Can you work these out from the model? Positions are in its coordinate system, mm. Give positions to 0.01 mm unless a question says otherwise; leave off trailing zeros. Write each loop counter-clockwise with the first axis right and the second up, starting at its lowest first coordinate (ties: lowest second). Pieces come first, ordered by that corner, then holes. Notation, with made-up numbers: M 18,47.5 L 66,47.5 A20 cw 66,78.5 Z; hole C 73,86.25 d11. An arc over 180 degrees is marked long. Answer as CSV lines item,"result". Start each with the question number.
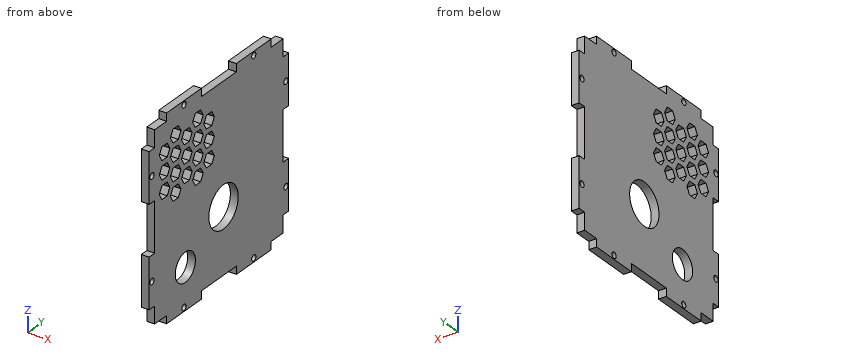
```python
from build123d import *

# Parameters (mm, degrees)
CROQUIS1_W                 = 70
CROQUIS1_H                 = 70
SALIENTE_EXTRUIR1_DEPTH    = 1.5
CROQUIS2_W                 = 19
CROQUIS2_H                 = 3
CROQUIS2_R                 = 1.15
SALIENTE_EXTRUIR2_DEPTH    = 1.5
MATRIZL1_COUNT             = 2
MATRIZL1_PITCH             = 38
SIMETR_A1_COPY_1_SKETCH_W  = 19
SIMETR_A1_COPY_1_SKETCH_H  = 3
SIMETR_A1_COPY_1_SKETCH_R  = 1.15
SIMETR_A1_COPY_1_DEPTH     = 1.5
CROQUIS5_W                 = 3
CROQUIS5_H                 = 19
CROQUIS5_R                 = 1.15
SALIENTE_EXTRUIR3_DEPTH    = 1.5
MATRIZL2_COUNT             = 2
MATRIZL2_PITCH             = 38
SIMETR_A2_COPY_1_SKETCH_W  = 3
SIMETR_A2_COPY_1_SKETCH_H  = 19
SIMETR_A2_COPY_1_SKETCH_R  = 1.15
SIMETR_A2_COPY_1_DEPTH     = 1.5
CORTAR_EXTRUIR2_DEPTH      = 54.761045377
CORTAR_EXTRUIR2_DEPTH_BACK = 54.761045377
CROQUIS4_R                 = 5.5
CORTAR_EXTRUIR3_DEPTH      = 54.761045377
CORTAR_EXTRUIR3_DEPTH_BACK = 54.761045377
CROQUIS6_R                 = 8
CORTAR_EXTRUIR7_DEPTH      = 54.761045377
CORTAR_EXTRUIR7_DEPTH_BACK = 54.761045377
PATR_N_START               = -1.5
PATR_N_DE_RAYADO3_DEPTH    = 3


# Read off the part's stored shape, not the designer's step: Patrón de rayado3
with BuildPart() as part:
    # Croquis1 → Saliente-Extruir1 (new, symmetric)
    with BuildSketch(Plane(origin=(0, 0, 0), x_dir=(0, 0, -1), z_dir=(1, 0, 0))):
        Rectangle(CROQUIS1_W, CROQUIS1_H)
    extrude(amount=SALIENTE_EXTRUIR1_DEPTH, both=True)

    # Croquis2 → Saliente-Extruir2 (add, symmetric)
    with BuildSketch(Plane(origin=(0, 0, 0), x_dir=(0, 0, -1), z_dir=(1, 0, 0))):
        with Locations((-19, 36.5)):
            Rectangle(CROQUIS2_W, CROQUIS2_H)
        with Locations((-19, 36.5)):
            Circle(CROQUIS2_R, mode=Mode.SUBTRACT)
    saliente_extruir2 = extrude(amount=SALIENTE_EXTRUIR2_DEPTH, both=True)

    # MatrizL1: Saliente-Extruir2 ×2
    with Locations(*[(0, 0, -i * MATRIZL1_PITCH) for i in range(1, MATRIZL1_COUNT)]):
        add(saliente_extruir2)

    # Simetría1: Saliente-Extruir2 across plane
    add(saliente_extruir2.mirror(Plane.ZX))

    # Simetría1 copy 1 sketch → Simetría1 copy 1 (add, symmetric)
    with BuildSketch(Plane(origin=(0, 0, -38), x_dir=(0, 0, -1), z_dir=(1, 0, 0))):
        with Locations((-19, -36.5)):
            Rectangle(SIMETR_A1_COPY_1_SKETCH_W, SIMETR_A1_COPY_1_SKETCH_H)
        with Locations((-19, -36.5)):
            Circle(SIMETR_A1_COPY_1_SKETCH_R, mode=Mode.SUBTRACT)
    extrude(amount=SIMETR_A1_COPY_1_DEPTH, both=True)

    # Croquis5 → Saliente-Extruir3 (add, symmetric)
    with BuildSketch(Plane(origin=(0, 0, 0), x_dir=(0, 0, -1), z_dir=(1, 0, 0))):
        with Locations((-36.5, 19)):
            Rectangle(CROQUIS5_W, CROQUIS5_H)
        with Locations((-36.5, 19)):
            Circle(CROQUIS5_R, mode=Mode.SUBTRACT)
    saliente_extruir3 = extrude(amount=SALIENTE_EXTRUIR3_DEPTH, both=True)

    # MatrizL2: Saliente-Extruir3 ×2
    with Locations(*[(0, -i * MATRIZL2_PITCH, 0) for i in range(1, MATRIZL2_COUNT)]):
        add(saliente_extruir3)

    # Simetría2: Saliente-Extruir3 across plane
    add(saliente_extruir3.mirror(Plane.XY))

    # Simetría2 copy 1 sketch → Simetría2 copy 1 (add, symmetric)
    with BuildSketch(Plane(origin=(0, -38, 0), x_dir=(0, 0, 1), z_dir=(1, 0, 0))):
        with Locations((-36.5, -19)):
            Rectangle(SIMETR_A2_COPY_1_SKETCH_W, SIMETR_A2_COPY_1_SKETCH_H)
        with Locations((-36.5, -19)):
            Circle(SIMETR_A2_COPY_1_SKETCH_R, mode=Mode.SUBTRACT)
    extrude(amount=SIMETR_A2_COPY_1_DEPTH, both=True)

    # Croquis4 → Cortar-Extruir2 (cut, two sides: drawn at the far end of the back side and taken through both)
    with BuildSketch(Plane(origin=(0, 0, 0), x_dir=(0, 0, -1), z_dir=(1, 0, 0)).offset(-CORTAR_EXTRUIR2_DEPTH_BACK)):
        with Locations((22.355, -18.3)):
            Circle(CROQUIS4_R)
    extrude(amount=CORTAR_EXTRUIR2_DEPTH + CORTAR_EXTRUIR2_DEPTH_BACK, mode=Mode.SUBTRACT)

    # Croquis6 → Cortar-Extruir3 (cut, two sides: drawn at the far end of the back side and taken through both)
    with BuildSketch(Plane(origin=(0, 0, 0), x_dir=(0, 0, -1), z_dir=(1, 0, 0)).offset(-CORTAR_EXTRUIR3_DEPTH_BACK)):
        with Locations((10.355, 2.5)):
            Circle(CROQUIS6_R)
    extrude(amount=CORTAR_EXTRUIR3_DEPTH + CORTAR_EXTRUIR3_DEPTH_BACK, mode=Mode.SUBTRACT)

    # Croquis11 → Cortar-Extruir7 (cut, two sides: drawn at the far end of the back side and taken through both)
    with BuildSketch(Plane(origin=(0, 0, 0), x_dir=(0, 0, -1), z_dir=(1, 0, 0)).offset(-CORTAR_EXTRUIR7_DEPTH_BACK)):
        Polygon((-20, -16.056624327), (-20, -18.943375673), (-17.5, -20.386751346), (-15, -18.943375673), (-15, -16.056624327), (-17.5, -14.613248654), align=None)
    extrude(amount=CORTAR_EXTRUIR7_DEPTH + CORTAR_EXTRUIR7_DEPTH_BACK, mode=Mode.SUBTRACT)

    # Patrón de rayado3 outline → Patrón de rayado3 (cut)
    with BuildSketch(Plane.YZ.offset(PATR_N_START)):
        Polygon((-20.675426481, 7), (-22.118802154, 9.5), (-25.005553499, 9.5), (-26.448929172, 7), (-25.005553499, 4.5), (-22.118802154, 4.5), align=None)
        Polygon((-8.551070828, 7), (-9.994446501, 9.5), (-12.881197846, 9.5), (-14.324573519, 7), (-12.881197846, 4.5), (-9.994446501, 4.5), align=None)
        Polygon((-22.118802154, 25.5), (-20.675426481, 28), (-22.118802154, 30.5), (-25.005553499, 30.5), (-26.448929172, 28), (-25.005553499, 25.5), align=None)
        Polygon((-12.881197846, 25.5), (-9.994446501, 25.5), (-8.551070828, 28), (-9.994446501, 30.5), (-12.881197846, 30.5), (-14.324573519, 28), align=None)
        Polygon((-32.511106999, 17.5), (-31.067731326, 15), (-28.18097998, 15), (-26.737604307, 17.5), (-28.18097998, 20), (-31.067731326, 20), align=None)
        Polygon((-8.262395693, 17.5), (-6.81902002, 15), (-3.932268674, 15), (-2.488893001, 17.5), (-3.932268674, 20), (-6.81902002, 20), align=None)
        Polygon((-16.056624327, 8), (-14.613248654, 10.5), (-16.056624327, 13), (-18.943375673, 13), (-20.386751346, 10.5), (-18.943375673, 8), align=None)
        Polygon((-22.118802154, 18.5), (-20.675426481, 21), (-22.118802154, 23.5), (-25.005553499, 23.5), (-26.448929172, 21), (-25.005553499, 18.5), align=None)
        Polygon((-12.881197846, 18.5), (-9.994446501, 18.5), (-8.551070828, 21), (-9.994446501, 23.5), (-12.881197846, 23.5), (-14.324573519, 21), align=None)
        Polygon((-8.262395693, 10.5), (-6.81902002, 8), (-3.932268674, 8), (-2.488893001, 10.5), (-3.932268674, 13), (-6.81902002, 13), align=None)
        Polygon((-32.511106999, 10.5), (-31.067731326, 8), (-28.18097998, 8), (-26.737604307, 10.5), (-28.18097998, 13), (-31.067731326, 13), align=None)
        Polygon((-22.118802154, 11.5), (-20.675426481, 14), (-22.118802154, 16.5), (-25.005553499, 16.5), (-26.448929172, 14), (-25.005553499, 11.5), align=None)
        Polygon((-28.18097998, 22), (-26.737604307, 24.5), (-28.18097998, 27), (-31.067731326, 27), (-32.511106999, 24.5), (-31.067731326, 22), align=None)
        Polygon((-18.943375673, 22), (-16.056624327, 22), (-14.613248654, 24.5), (-16.056624327, 27), (-18.943375673, 27), (-20.386751346, 24.5), align=None)
        Polygon((-14.324573519, 14), (-12.881197846, 11.5), (-9.994446501, 11.5), (-8.551070828, 14), (-9.994446501, 16.5), (-12.881197846, 16.5), align=None)
        Polygon((-8.262395693, 24.5), (-6.81902002, 22), (-3.932268674, 22), (-2.488893001, 24.5), (-3.932268674, 27), (-6.81902002, 27), align=None)
    extrude(amount=PATR_N_DE_RAYADO3_DEPTH, mode=Mode.SUBTRACT)


solid = part.part
```
1) I want a section at A-A, the plane y = -36.5. Please give me the cut outline in (x, z), then the cut area to 3 significant figures.
2) I want a section at D-D, the plane z = -22. Please give me the cut outline in (x, y).
3) I need wall thicknesses on L1, parallel to Z at x = -0.5, y = -30.5; L2, parallel to Y at x = -0.5, z = -19; L3, parallel to Z at x = 1, y = -24.5. Which ranges of each line are inside material? Lowest first, please. Write a range as from..to.
4) I'm going to push flat-ended pins straight in: P1, Ø0.9, axis at x = 0.5, z = 36.5, coming from the -Y side; P2, Ø0.9, axis at x = 0, y = 31.5, coming from the -Z side. Where does each tip first touch, or does it pass through?
5) I want a section at C-C, the plane y = 2.5. Please give me the cut outline in (x, z) (3 decimals), then the cut area to 3 significant figures.
Values found:
1,outline,"M -1.5,-28.5 L 1.5,-28.5 L 1.5,-20.15 L -1.5,-20.15 Z; M -1.5,-17.85 L 1.5,-17.85 L 1.5,-9.5 L -1.5,-9.5 Z; M -1.5,9.5 L 1.5,9.5 L 1.5,17.85 L -1.5,17.85 Z; M -1.5,20.15 L 1.5,20.15 L 1.5,28.5 L -1.5,28.5 Z"
1,area,"100 mm²"
2,outline,"M -1.5,-38 L 1.5,-38 L 1.5,-23.79 L -1.5,-23.79 Z; M -1.5,-12.81 L 1.5,-12.81 L 1.5,38 L -1.5,38 Z"
3,L1,"z = -35..8, 13..15, 20..22, 27..35"
3,L2,"y = -38..-37.65, -35.35..-22.66, -13.94..35.35, 37.65..38"
3,L3,"z = -38..4.5, 9.5..11.5, 16.5..18.5, 23.5..25.5, 30.5..38"
4,P1,"stops at y = -28.5"
4,P2,"stops at z = -35"
5,outline,"M -1.5,-35 L 1.5,-35 L 1.5,-18.355 L -1.5,-18.355 Z; M -1.5,-2.355 L 1.5,-2.355 L 1.5,35 L -1.5,35 Z"
5,area,"162 mm²"
